from build123d import *

# Parameters (mm, degrees)
F1_R     = 30.580116
F1_R_2   = 26.414557
F2_DEPTH = 42.605285
F3_R     = 38.1
F4_DEPTH = 12.7
F5_R     = 23.348027
F6_DEPTH = 25.4


with BuildPart() as f2:
    # F1 (on offset) → F2 (new body)
    with BuildSketch(Plane.XY.offset(-64.257657)):
        Circle(F1_R)
        Circle(F1_R_2, mode=Mode.SUBTRACT)
    extrude(amount=F2_DEPTH)

    # F3 (on offset) → F4 (join)
    with BuildSketch(Plane.XY.offset(-64.257657)):
        Circle(F3_R)
    extrude(amount=-F4_DEPTH)

    # F5 (on face) → F6 (cut)
    with BuildSketch(Plane.XY.offset(-64.257657)):
        Circle(F5_R)
    extrude(amount=-F6_DEPTH, mode=Mode.SUBTRACT)


solid = f2.part
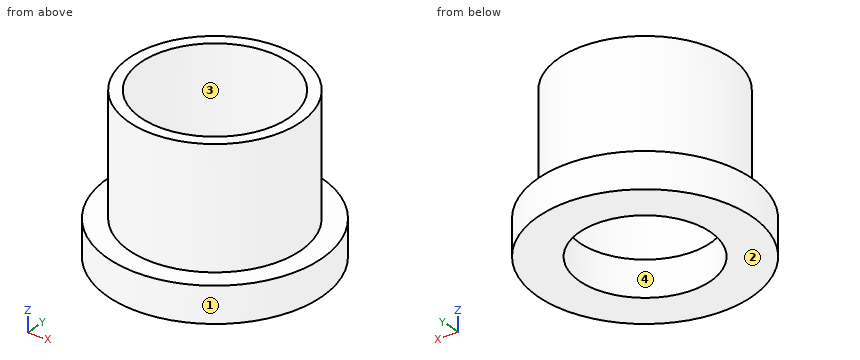
The listing builds one solid part. Answer for the finished solid, in the listing's coordinates (mm). Face numbers are marked on the shaded views. Coordinates: 2 decimals unless noted, no trailing zeros. Write each loop counter-clockwise with the first axis right and the second up, starting at its lowest first coordinate (ties: lowest second). Pieces come first, ordered by that corner, then holes. Notation, with made-up numbers: (54, -7.75) - (75, -7.75) arc R26 cw to (75, 26.25) - close; hole circle Ø4 at (33.25, -32.75). An arc over 180 degrees is marked (long way). Answer as CSV lines item,"result".
1. Straight lines are drawn through the part: line 1 (X direction, y = -0.5, z = -71); line 2 (Y direction, x = 0, z = -32.5); line 3 (Y direction, x = 0, z = -68). For each, find the intervals that lie inside material, in ascending order. Write a range as [from, to].
Computed values:
line 1,"x = [-38.1, -23.34], [23.34, 38.1]"
line 2,"y = [-30.58, -26.41], [26.41, 30.58]"
line 3,"y = [-38.1, -23.35], [23.35, 38.1]"
2. Find section A-A (x = 0). Give the vertices of the cut face in (y, z).
Computed values:
outline,"(-38.1, -76.96) - (-23.35, -76.96) - (-23.35, -64.26) - (-26.41, -64.26) - (-26.41, -21.65) - (-30.58, -21.65) - (-30.58, -64.26) - (-38.1, -64.26) - close; (23.35, -76.96) - (38.1, -76.96) - (38.1, -64.26) - (30.58, -64.26) - (30.58, -21.65) - (26.41, -21.65) - (26.41, -64.26) - (23.35, -64.26) - close"
3. Given P1, Ø12, axis at x = 2.5, z = -42.5, coming from the +Y side; P2, Ø12, axis at y = -7.5, z = -69.5, coming from the -X side; P3, Ø1, axis at y = 27.5, z = -65.5, coming from the -X side; P4, Ø8, axis at x = 12.5, y = 28, coming from the +Z side, each flat-ended and moving along its own axis, determine where each tip first touches the part or whether it passes through.
Computed values:
P1,"stops at y = 30.58"
P2,"stops at x = -38.07"
P3,"stops at x = -26.88"
P4,"stops at z = -21.65"
4. Find section D-D (z = -66). Give the vertices of the cut face in (x, y).
Computed values:
outline,"circle Ø76.2 at (0, 0); hole circle Ø46.7 at (0, 0)"
5. Determine the mould class of the marked faces 1, 2, 3 and 4 for opening direction Y: +Y half, -Y half, draft (parallel to the pull), parting line (faces both ways), or undercut.
Computed values:
face 1,"parting line"
face 2,"draft"
face 3,"undercut"
face 4,"undercut"
6. Find section C-C (z = -34.5). Give the vertices of the cut face in (x, y), plus the area to 3 significant figures.
Computed values:
outline,"circle Ø61.16 at (0, 0); hole circle Ø52.83 at (0, 0)"
area,"746 mm²"
